from build123d import *

# Parameters (mm, degrees)
F1_DEPTH = 57.1
F2_R     = 11
F3_DEPTH = 44.5
F4_R     = 3.05
F5_DEPTH = 7.8
F6_R     = 6


with BuildPart() as f1:
    # F0 (on Top) → F1 (new body)
    with BuildSketch(Plane.XY):
        Polygon((-31.75, 44.5), (-31.75, 0), (26.95, 0), (31.75, 44.5), align=None)
    extrude(amount=F1_DEPTH)

    # F2 (on face) → F3 (cut, through all)
    with BuildSketch(Plane.XZ):
        with Locations((0, 40)):
            Circle(F2_R)
    extrude(amount=-F3_DEPTH, mode=Mode.SUBTRACT)

    # F4 (on face) → F5 (cut)
    with BuildSketch(Plane(origin=(0, 0, 0), x_dir=(1, 0, 0), z_dir=(0, 0, -1))):
        with Locations((0, -5.18)):
            Circle(F4_R)
    extrude(amount=-F5_DEPTH, mode=Mode.SUBTRACT)

    # F6
    f6_edges = [f1.edges().sort_by_distance(p)[0] for p in [
        (-31.75, 0, 28.55),
        (-31.75, 44.5, 28.55),
        (26.95, 0, 28.55),
        (31.75, 44.5, 28.55),
    ]]
    fillet(f6_edges, radius=F6_R)


solid = f1.part
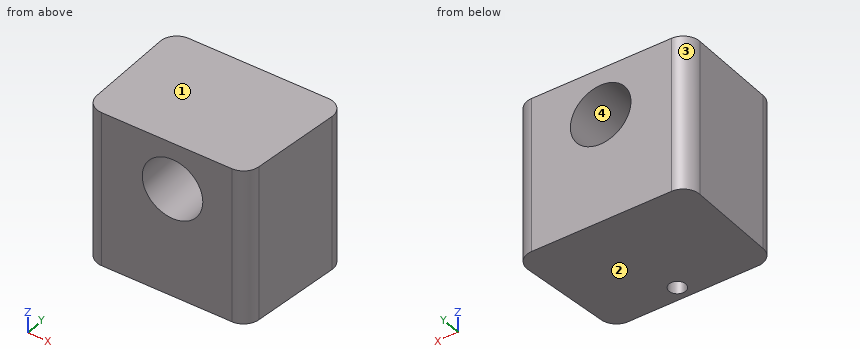
CAD build for the part. Positions are in the model's coordinates, mm. Face numbers are marked on the shaded views. Round coordinates to 2 decimals unless told otherwise and drop trailing zeros. Write each loop counter-clockwise with the first axis right and the second up, starting at its lowest first coordinate (ties: lowest second). Pieces come first, ordered by that corner, then holes.
(1) Slice it at B-B, the plane x = 0. Write the cut outline in (y, z), and give its area (3 significant figures).
(2) Drop flat-ended pins along their axis: P1, Ø20, axis at x = 0, z = 40, coming from the +Y side; P2, Ø4, axis at x = -11, y = 18.5, coming from the -Z side; P3, Ø4, axis at y = 18.5, z = 9.5, coming from the +X side; P4, Ø5, axis at x = 0, y = 5.18, coming from the -Z side. Give the stop position or say it passes through.
(3) Slice it at A-A, the plane z = 40. Write the cut outline in (x, y).
(4) Probe line 1 along Z through (x, y) = (0, 26); line 2 along Z through (x, y) = (3.5, 14); line 3 along X through (y, z) = (5, 4). List the from-to ranges inside material, lowest first.
(5) Slice it at C-C, the plane z = 52. Write the cut outline in (x, y).
(6) Mould opens along Z. For the marked faces 1, 2, 3 and 4 say: pulls with the +Z half, pulls with the -Z half, needs draft (parallel to the pull), parting line crosses it, or undercut.
(7) Slice it at D-D, the plane y = 30. Write the cut outline in (x, z).
From the geometry:
1. outline: (0, 0) - (2.13, 0) - (2.13, 7.8) - (8.23, 7.8) - (8.23, 0) - (44.5, 0) - (44.5, 29) - (0, 29) - close; (0, 51) - (44.5, 51) - (44.5, 57.1) - (0, 57.1) - close
1. area: 1,510 mm2
2. P1: passes through
2. P2: stops at z = 0
2. P3: stops at x = 29.16
2. P4: stops at z = 7.8
3. outline: (-31.75, 6) arc R6 ccw to (-25.75, 0) - (-11, 0) - (-11, 44.5) - (-25.75, 44.5) arc R6 ccw to (-31.75, 38.5) - close; (11, 0) - (21.56, 0) arc R6 ccw to (27.53, 5.36) - (31.03, 37.86) arc R6 ccw to (25.07, 44.5) - (11, 44.5) - close
4. line 1: z = 0 to 29, 51 to 57.1
4. line 2: z = 0 to 29.57, 50.43 to 57.1
4. line 3: x = -31.67 to -3.04, 3.04 to 27.48
5. outline: (-31.75, 6) arc R6 ccw to (-25.75, 0) - (21.56, 0) arc R6 ccw to (27.53, 5.36) - (31.03, 37.86) arc R6 ccw to (25.07, 44.5) - (-25.75, 44.5) arc R6 ccw to (-31.75, 38.5) - close
6. face 1: pulls with the +Z half
6. face 2: pulls with the -Z half
6. face 3: needs draft
6. face 4: undercut
7. outline: (-31.75, 0) - (30.19, 0) - (30.19, 57.1) - (-31.75, 57.1) - close; hole circle Ø22 at (0, 40)
